Source: CAD feature listing. Evaluate the final solid. Frame: model axes, mm. Face numbers are marked on the shaded views. Coordinates: 2 decimals unless noted, no trailing zeros. Loops run counter-clockwise (first coordinate to the right, second up) from the corner with the lowest first, then second, coordinate; pieces in that order, holes last.
Item 1: Section query D-D, the plane z = -11.5. Return the cut outline in (x, y), then the cut area to 3 significant figures.
Item 2: Section query A-A, the plane z = 0. Return the cut outline in (x, y).
Item 3: Section query B-B, the plane y = -31. Return the cut outline in (x, z).
Item 4: Pin query (flat end, axial travel): pin 1 Ø1.5 at (x, y) = (-0.5, -5.5) entering from -Z; pin 2 Ø1 at (x, y) = (-6, -39) entering from -Z. Return the tip coordinate at first contact, or that it passes through.
Item 5: Pull-direction query (Z, two-part tool) for the marked faces 1, 2, 3 and 4; classes: +Z half, -Z half, draft (parallel to the pull), parting line (faces both ways), or undercut.
Item 6: Line query: probe 1 along Y at (x, z) = (-10.75, -6.5); probe 2 along Z at (x, y) = (-1, -22); probe 3 along X at (y, z) = (-51, -3). Output: solid intervals per line, ascending.
Item 7: Section query C-C, the plane x = 2.75. Return the cut outline in (y, z).
```python
from build123d import *

# Parameters (mm, degrees)
F0_R     = 6.35
F1_DEPTH = 69.85
F2_R     = 6.35
F3_DEPTH = 6.35


with BuildPart() as f1:
    # F0 (on Front) → F1 (new body)
    with BuildSketch(Plane.XZ):
        Circle(F0_R)
    extrude(amount=F1_DEPTH)

    # F2 (on face) → F3 (join)
    with BuildSketch(Plane(origin=(0, 0, 0), x_dir=(-1, 0, 0), z_dir=(0, 1, 0))):
        Polygon((14.4728282073, 7.9192246264), (0.3781643989, 16.4934492053), (-14.0946638083, 8.5742245789), (-14.4728282073, -7.9192246264), (-0.3781643989, -16.4934492053), (14.0946638083, -8.5742245789), align=None)
        Circle(F2_R, mode=Mode.SUBTRACT)
        Circle(F2_R)
    extrude(amount=F3_DEPTH)


solid = f1.part
```
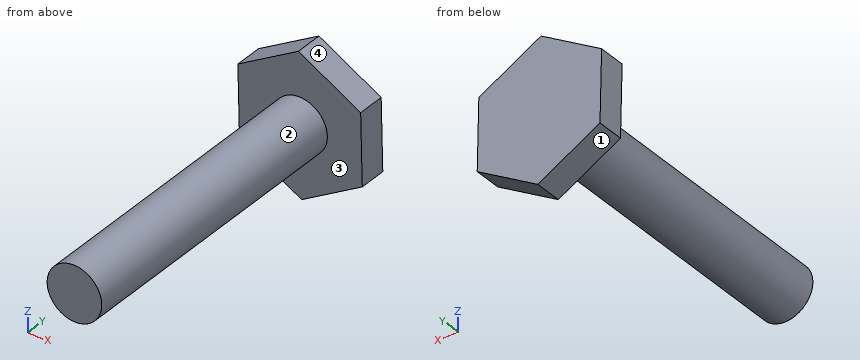
Verdict:
1. outline: (-8.75, 0) - (8.59, 0) - (8.59, 6.35) - (-8.75, 6.35) - close
1. area: 110 mm2
2. outline: (-14.29, 0) - (-6.35, 0) - (-6.35, -69.85) - (6.35, -69.85) - (6.35, 0) - (14.29, 0) - (14.29, 6.35) - (-14.29, 6.35) - close
3. outline: circle Ø12.7 at (0, 0)
4. pin 1: stops at z = -6.35
4. pin 2: stops at z = -3.17
5. face 1: -Z half
5. face 2: parting line
5. face 3: draft
5. face 4: +Z half
6. probe 1: y = 0 to 6.35
6. probe 2: z = -6.27 to 6.27
6. probe 3: x = -5.6 to 5.6
7. outline: (-69.85, -5.72) - (0, -5.72) - (0, -15.05) - (6.35, -15.05) - (6.35, 14.78) - (0, 14.78) - (0, 5.72) - (-69.85, 5.72) - close
